Geometry check sheet. Reference: the model listing, model coordinates, mm. Face numbers are marked on the shaded views. A direction names the side the tool comes from. Coordinates: 2 decimals unless noted, no trailing zeros. Write each loop counter-clockwise with the first axis right and the second up, starting at its lowest first coordinate (ties: lowest second). Pieces come first, ordered by that corner, then holes. Notation, with made-up numbers: (49.25, 41) -> (94.25, 41) arc R36 ccw to (94.25, 78) -> close; hole circle Ø11 at (6.5, 39.25). An arc over 180 degrees is marked (long way). Answer in a Markdown table with one row per item. Add a question column.
Q1. Section check D-D, the plane y = -22.5. Record the boundary of the cut face in (x, z).
Q2. Gauge pin test, flat ends, axial feed: P1, Ø7.5, axis at y = -4, z = 29, coming from the +X side; P2, Ø9, axis at x = -8.5, z = 46.5, coming from the -Y side; P3, Ø2, axis at x = 4.5, y = 8.5, coming from the +Z side; P4, Ø1, axis at y = 4.5, z = 55.5, coming from the +X side. Record the tip position at first contact, or that the pin passes through.
Q3. Section check C-C, the plane x = -14.5. Record the boundary of the cut face in (y, z).
Q4. Section check B-B, the plane y = 13. Record the boundary of the cut face in (x, z), and give its area (3 significant figures).
Q5. Thickness scan on line 1 (X direction, y = -15.5, z = 57.5); line 2 (Y direction, x = -9.5, z = 40); line 3 (Y direction, x = -5, z = 32.5). Record the ranges inside material, lowest first.
Q6. Release check for a two-part mould opening along X. For the marked faces 1, 2 and 3 record: pulls with the +X half, pulls with the -X half, needs draft (parallel to the pull), parting line crosses it, or undercut.
Q7. Section check A-A, the plane z = 18.5. Record the boundary of the cut face in (x, y).
Q8. Tool access check on the marked faces 4 and 5. Record the directions out of +Z, -Z, +X, -X, +Y, -Y that give a thin tool (end or side, any length) a straight path to the whole face; none if there is none.
```python
from build123d import *

# Parameters (mm, degrees)
BOSS_EXTRUDE1_DEPTH = 70


with BuildPart() as part:
    # Sketch2 → Boss-Extrude1 (new body)
    with BuildSketch(Plane.XY):
        with BuildLine():
            ThreePointArc((21.020681104, 22.985087501), (25.748004826, 19.613709748), (24.100290936, 14.04605167))
            Line((24.100290936, 14.04605167), (-30.899709064, -28.95394833))
            ThreePointArc((-30.899709064, -28.95394833), (-36.170431723, -29.509244994), (-38.979318896, -25.014912499))
            Line((-38.979318896, -25.014912499), (-38.979318896, 17.985087501))
            ThreePointArc((-38.979318896, 17.985087501), (-37.514852802, 21.520621407), (-33.979318896, 22.985087501))
            Line((-33.979318896, 22.985087501), (21.020681104, 22.985087501))
        make_face()
        with BuildLine():
            ThreePointArc((6.245861273, 11.998107897), (4.781395179, 15.533641803), (1.245861273, 16.998107897))
            Line((1.245861273, 16.998107897), (-29.453101677, 16.998107897))
            ThreePointArc((-29.453101677, 16.998107897), (-32.988635583, 15.533641803), (-34.453101677, 11.998107897))
            Line((-34.453101677, 11.998107897), (-34.453101677, -13.737840514))
            ThreePointArc((-34.453101677, -13.737840514), (-31.644214504, -18.232173009), (-26.373491845, -17.676876345))
            Line((-26.373491845, -17.676876345), (4.325471105, 6.324131052))
            ThreePointArc((4.325471105, 6.324131052), (5.740193768, 8.072054056), (6.245861273, 10.263166883))
            Line((6.245861273, 10.263166883), (6.245861273, 11.998107897))
        make_face(mode=Mode.SUBTRACT)
    extrude(amount=BOSS_EXTRUDE1_DEPTH)


solid = part.part
```
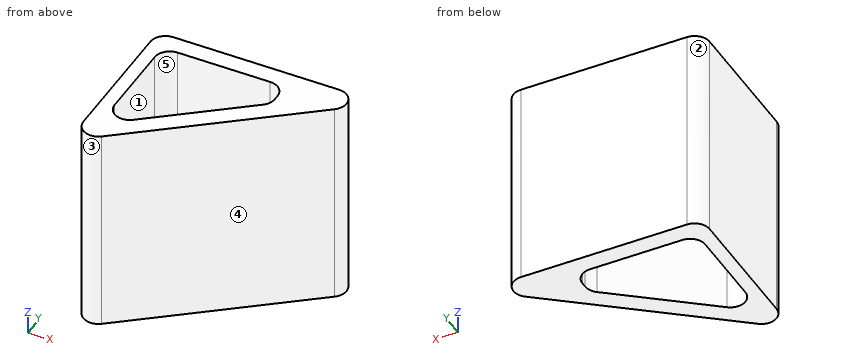
Calculated:
| question | item | result |
|---|---|---|
| 1 | outline | (-38.98, 0) -> (-22.64, 0) -> (-22.64, 70) -> (-38.98, 70) -> close |
| 2 | P1 | stops at x = 5.81 |
| 2 | P2 | stops at y = -14.96 |
| 2 | P3 | passes through |
| 2 | P4 | stops at x = 12.53 |
| 3 | outline | (-16.13, 0) -> (-8.39, 0) -> (-8.39, 70) -> (-16.13, 70) -> close; (17, 0) -> (22.99, 0) -> (22.99, 70) -> (17, 70) -> close |
| 4 | outline | (-38.98, 0) -> (-34.35, 0) -> (-34.35, 70) -> (-38.98, 70) -> close; (6.14, 0) -> (22.76, 0) -> (22.76, 70) -> (6.14, 70) -> close |
| 4 | area | 1,490 mm² |
| 5 | line 1 | x = -38.98 to -34.13, -23.59 to -13.69 |
| 5 | line 2 | y = -12.22 to -4.48, 17 to 22.99 |
| 5 | line 3 | y = -8.71 to -0.97, 17 to 22.99 |
| 6 | face 1 | undercut |
| 6 | face 2 | pulls with the -X half |
| 6 | face 3 | parting line crosses it |
| 7 | outline | (-38.98, -25.01) arc R5 ccw to (-30.9, -28.95) -> (24.1, 14.05) arc R5 ccw to (21.02, 22.99) -> (-33.98, 22.99) arc R5 ccw to (-38.98, 17.99) -> close; hole (-34.45, -13.74) arc R5 ccw to (-26.37, -17.68) -> (4.33, 6.32) arc R5 ccw to (6.25, 10.26) -> (6.25, 12) arc R5 ccw to (1.25, 17) -> (-29.45, 17) arc R5 ccw to (-34.45, 12) -> close |
| 8 | face 4 | +Z, -Z, +X, -Y |
| 8 | face 5 | +Z, -Z |
